from build123d import *

# Parameters (mm, degrees)
ESQUISSE2_R             = 3
BOSS_EXTRU_1_DEPTH      = 20
CONG_1_R                = 0.5
ESQUISSE3_R             = 2.8
ENL_V_MAT_EXTRU_1_DEPTH = 0.2
ESQUISSE4_R             = 1.25
BOSS_EXTRU_2_DEPTH      = 20.2


with BuildPart() as part:
    # Esquisse2 → Boss.-Extru.1 (new body)
    with BuildSketch(Plane.XY):
        Circle(ESQUISSE2_R)
    extrude(amount=BOSS_EXTRU_1_DEPTH)

    # Congé1
    cong_1_edges = [part.edges().sort_by_distance(p)[0] for p in [
        (-3, 0, 0),
    ]]
    fillet(cong_1_edges, radius=CONG_1_R)

    # Esquisse3 → Enlèv. mat.-Extru.1 (cut)
    with BuildSketch(Plane.XY.offset(20)):
        Circle(ESQUISSE3_R)
    extrude(amount=-ENL_V_MAT_EXTRU_1_DEPTH, mode=Mode.SUBTRACT)

    # Esquisse4 → Boss.-Extru.2 (add)
    with BuildSketch(Plane.XY.offset(19.8)):
        with Locations((-1.4, 0)):
            Circle(ESQUISSE4_R)
        with Locations((1.4, 0)):
            Circle(ESQUISSE4_R)
    extrude(amount=BOSS_EXTRU_2_DEPTH)


solid = part.part
Check sheet for the modelled part. Datum: model origin and axes. Units: mm. A direction names the side the tool comes from. Give positions to 0.01 mm unless a question says otherwise; leave off trailing zeros. Loops run counter-clockwise (first coordinate to the right, second up) from the corner with the lowest first, then second, coordinate; pieces in that order, holes last. Notation, with made-up numbers: M 65.5,46.25 L 120.5,46.25 A35 cw 120.5,84.25 Z; hole C -32.75,-13.75 d1. An arc over 180 degrees is marked long. Use a Markdown table: item, result. Add a question column.
Q1. Tool access check on faces 1 (the flat face through (1, 0, 40)), 2 (the cylindrical face through (2.555, -0.479, 29.759)). Record the directions out of +Z, -Z, +X, -X, +Y, -Y that give a thin tool (end or side, any length) a straight path to the whole face; none if there is none.
Q2. Go/stop test with a flat-tipped pin: pin 1 (2 mm diameter, centred on x = -1, z = 27.5, fed in from -Y). Record where the tip stops, or that it passes through.
Q3. Mould release check, pull along X, two halves, no side actions. Record for faces 3 (the cylindrical face through (-0.21, 0.38, 29.76)), 4 (the flat face through (0, 0, 0)), 5 (the cylindrical face through (-3, 0, 10)): pulls with the +X half, pulls with the -X half, needs draft (parallel to the pull), parting line crosses it, or undercut.
Q4. Sectioned sample at B-B, the plane z = 21. Record the cut outline in (x, y).
Q5. Sectioned sample at C-C, the plane z = 12. Record the cut outline in (x, y).
Q6. Sectioned sample at A-A, the plane y = 0. Record the cut outline in (x, z), then the cut area to 3 significant figures.
Q7. Scan lines: line 1 along Y through (x, z) = (0, 19.9); line 2 along Z through (x, y) = (-0.1, -1.65); line 3 along X through (y, z) = (-2.7, 18). Record each from-to range of solid material in increasing order. Write a range as [from, to].
Verdict:
| question | item | result |
|---|---|---|
| 1 | face 1 | +Z, +X, -X, +Y, -Y |
| 1 | face 2 | +Z |
| 2 | pin 1 | y = -1.25 |
| 3 | face 3 | undercut |
| 3 | face 4 | needs draft |
| 3 | face 5 | parting line crosses it |
| 4 | outline | C -1.4,0 d2.5; C 1.4,0 d2.5 |
| 5 | outline | C 0,0 d6 |
| 6 | outline | M -3,0.5 A0.5 ccw -2.5,0 L 2.5,0 A0.5 ccw 3,0.5 L 3,20 L 2.8,20 L 2.8,19.8 L 2.65,19.8 L 2.65,40 L 0.15,40 L 0.15,19.8 L -0.15,19.8 L -0.15,40 L -2.65,40 L -2.65,19.8 L -2.8,19.8 L -2.8,20 L -3,20 Z |
| 6 | area | 220 mm^2 |
| 7 | line 1 | [-3, -2.8], [2.8, 3] |
| 7 | line 2 | [0, 19.8] |
| 7 | line 3 | [-1.31, 1.31] |
